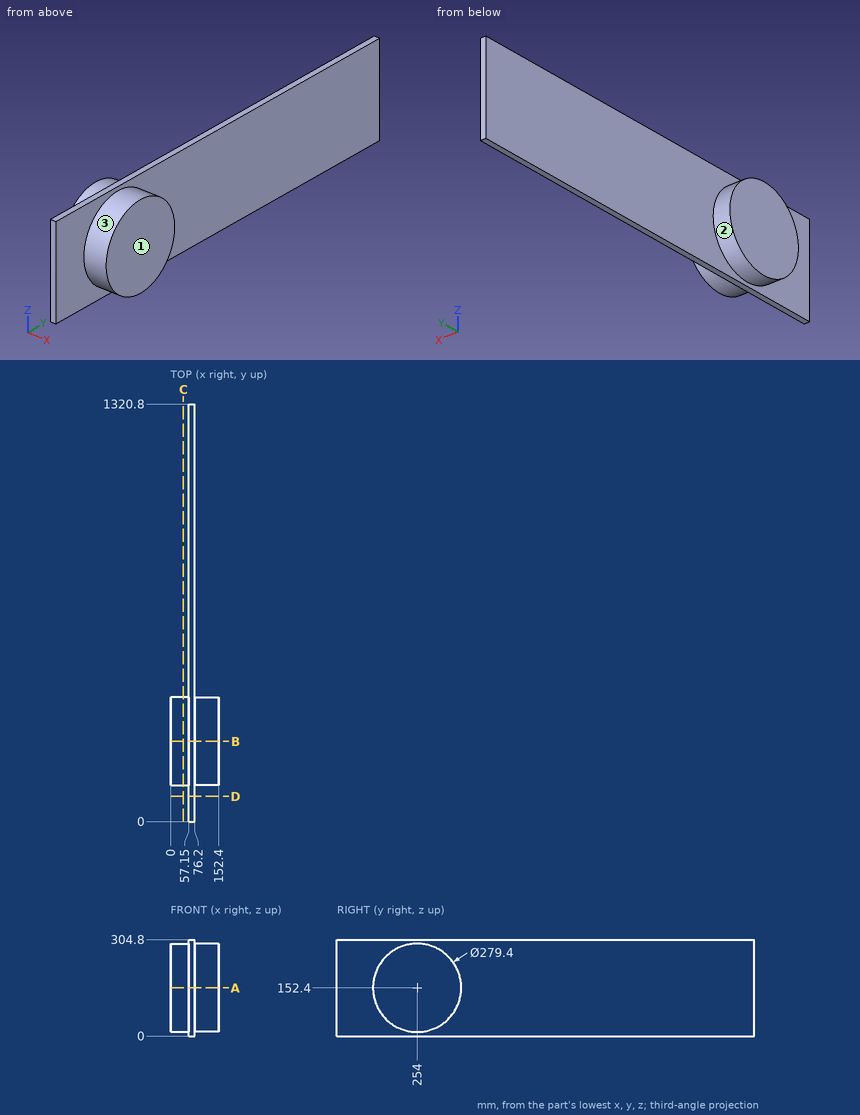
Source: three-view drawing plus pictorial views. Frame: mm from the lowest corner of the part. A direction names the side the tool comes from. Give positions to 0.01 mm unless a question says otherwise; leave off trailing zeros. Order: outer loops, then holes, each group sorted by start corner. A loop starts at its lowest first (then second) coordinate and runs counter-clockwise, first axis right, second up. Notation, with made-up numbers: (-36, 31.25) -> (-8, 31.25) arc R8 ccw to (-8, 38.25) -> close; hole circle Ø3 at (-9, -4). An arc over 180 degrees is marked (long way). Write each question's results on one line, items separated by ' | '. Start each with the question number.
Item 1: Set-up query: the marked faces 1, 2 and 3. Return all of +Z, -Z, +X, -X, +Y, -Y with unobstructed straight access to the full face (end or side cutting, diameter ignored); none if empty.
Item 2: Contact query for flat-ended pins moving along their axis: P1, Ø8, axis at x = 25, z = 244.5, coming from the -Y side; P2, Ø1.5, axis at x = 100.5, z = 105.5, coming from the -Y side; P3, Ø6, axis at y = 1040.5, z = 150.5, coming from the +X side. Output: stop coordinate, or through.
Item 3: Cut plane D-D on y = 80. Return the cut outline in (x, z).
Item 4: Cut plane A-A on z = 152.4. Return the cut outline in (x, y), then the cut area to 3 significant figures.
Item 5: Cut plane B-B on y = 254. Return the cut outline in (x, z).
Item 6: Cut plane C-C on x = 40.5. Return the cut outline in (y, z), then the cut area to 3 significant figures.
Item 7: Line query: line 1 (X direction, y = 776.5, z = 164); line 2 (Y direction, x = 78.5, z = 107.5); line 3 (Y direction, x = 6.5, z = 281). Output: solid intervals per line, ascending.
Established:
1) face 1: +Z, -Z, +X, +Y, -Y | face 2: -X | face 3: +X
2) P1: y = 145.58 | P2: y = 122.14 | P3: x = 76.2
3) outline: (57.15, 0) -> (76.2, 0) -> (76.2, 304.8) -> (57.15, 304.8) -> close
4) outline: (0, 114.3) -> (57.15, 114.3) -> (57.15, 0) -> (76.2, 0) -> (76.2, 114.3) -> (152.4, 114.3) -> (152.4, 393.7) -> (76.2, 393.7) -> (76.2, 1320.8) -> (57.15, 1320.8) -> (57.15, 393.7) -> (0, 393.7) -> close | area: 62,400 mm^2
5) outline: (0, 12.7) -> (57.15, 12.7) -> (57.15, 0) -> (76.2, 0) -> (76.2, 12.7) -> (152.4, 12.7) -> (152.4, 292.1) -> (76.2, 292.1) -> (76.2, 304.8) -> (57.15, 304.8) -> (57.15, 292.1) -> (0, 292.1) -> close
6) outline: circle Ø279.4 at (254, 152.4) | area: 61,300 mm^2
7) line 1: 57.15 to 76.2 | line 2: 121.71 to 386.29 | line 3: 199.43 to 308.57
